```python
from build123d import *

# Parameters (mm, degrees)
CROQUIS1_W              = 33.02
CROQUIS1_H              = 10.414
SALIENTE_EXTRUIR1_DEPTH = 0.5
CROQUIS2_R              = 2.5
CROQUIS2_R_2            = 2.35
CROQUIS2_R_3            = 0.9
CROQUIS2_R_4            = 0.7
CROQUIS2_W              = 2
CROQUIS2_H              = 2
SALIENTE_EXTRUIR2_DEPTH = 0.05
CORTAR_EXTRUIR1_START   = -30.1
CROQUIS3_R              = 2.35
CROQUIS3_R_2            = 0.7
CORTAR_EXTRUIR1_DEPTH   = 30.1
CROQUIS4_R              = 0.7
CORTAR_EXTRUIR2_DEPTH   = 40.1
CROQUIS5_W              = 22.32
CROQUIS5_H              = 8.014
SALIENTE_EXTRUIR3_DEPTH = 5
CROQUIS6_W              = 4.5
CROQUIS6_H              = 6.414
CORTAR_EXTRUIR3_DEPTH   = 1.5
CROQUIS7_R              = 3.5
CORTAR_EXTRUIR4_DEPTH   = 3
C_PULA1_FACE_RADIUS     = 3.5
C_PULA1_HEIGHT          = 3
C_PULA2_FACE_RADIUS     = 3.5
C_PULA2_HEIGHT          = 3.2
CROQUIS8_R              = 0.4
SALIENTE_EXTRUIR4_DEPTH = 0.05


with BuildPart() as part:
    # Croquis1 → Saliente-Extruir1 (new, symmetric)
    with BuildSketch(Plane.XY):
        Rectangle(CROQUIS1_W, CROQUIS1_H)
    extrude(amount=SALIENTE_EXTRUIR1_DEPTH, both=True)

    # Croquis2 → Saliente-Extruir2 (add)
    # profile 1 of 5: a face of its own
    with BuildSketch(Plane.XY.offset(0.5)):
        with Locations((-12.7, 0)):
            Circle(CROQUIS2_R)
        with Locations((-12.7, 0)):
            Circle(CROQUIS2_R_2, mode=Mode.SUBTRACT)
    # profile 2 of 5: a face of its own
    with BuildSketch(Plane.XY.offset(0.5)):
        with Locations((15.01, 3.707)):
            Circle(CROQUIS2_R_3)
        with Locations((15.01, 3.707)):
            Circle(CROQUIS2_R_4, mode=Mode.SUBTRACT)
    # profile 3 of 5: a face of its own
    with BuildSketch(Plane.XY.offset(0.5)):
        with Locations((15.01, 1.207)):
            Circle(CROQUIS2_R_3)
        with Locations((15.01, 1.207)):
            Circle(CROQUIS2_R_4, mode=Mode.SUBTRACT)
    # profile 4 of 5: a face of its own
    with BuildSketch(Plane.XY.offset(0.5)):
        with Locations((15.01, -1.293)):
            Circle(CROQUIS2_R_3)
        with Locations((15.01, -1.293)):
            Circle(CROQUIS2_R_4, mode=Mode.SUBTRACT)
    # profile 5 of 5: a face of its own
    with BuildSketch(Plane.XY.offset(0.5)):
        with Locations((15.01, -3.707)):
            Rectangle(CROQUIS2_W, CROQUIS2_H)
    extrude(amount=SALIENTE_EXTRUIR2_DEPTH)

    # Croquis3 → Cortar-Extruir1 (cut)
    with BuildSketch(Plane.XY.offset(0.5).offset(CORTAR_EXTRUIR1_START)):
        with Locations((-12.7, 0)):
            Circle(CROQUIS3_R)
        with Locations((15.01, 3.707)):
            Circle(CROQUIS3_R_2)
        with Locations((15.01, 1.207)):
            Circle(CROQUIS3_R_2)
        with Locations((15.01, -1.293)):
            Circle(CROQUIS3_R_2)
    extrude(amount=CORTAR_EXTRUIR1_DEPTH, mode=Mode.SUBTRACT)

    # Croquis4 → Cortar-Extruir2 (cut)
    with BuildSketch(Plane.XY.offset(0.55)):
        with Locations((15.01, -3.707)):
            Circle(CROQUIS4_R)
    extrude(amount=-CORTAR_EXTRUIR2_DEPTH, mode=Mode.SUBTRACT)

    # Croquis5 → Saliente-Extruir3 (add)
    with BuildSketch(Plane.XY.offset(0.5)):
        with Locations((2.15, 0)):
            Rectangle(CROQUIS5_W, CROQUIS5_H)
    extrude(amount=SALIENTE_EXTRUIR3_DEPTH)

    # Croquis6 → Cortar-Extruir3 (cut)
    with BuildSketch(Plane.XY.offset(5.5)):
        with Locations((2.15, 0)):
            Rectangle(CROQUIS6_W, CROQUIS6_H)
    extrude(amount=-CORTAR_EXTRUIR3_DEPTH, mode=Mode.SUBTRACT)

    # Croquis7 → Cortar-Extruir4 (cut)
    with BuildSketch(Plane.XY.offset(5.5)):
        with Locations((-4.8, 0)):
            Circle(CROQUIS7_R)
        with Locations((9.1, 0)):
            Circle(CROQUIS7_R)
    extrude(amount=-CORTAR_EXTRUIR4_DEPTH, mode=Mode.SUBTRACT)

    # Cúpula1: a dome of height H over a round flat face of radius A is a cap of a sphere of radius (A * A + H * H) / (2 * H)
    c_pula1_r = (C_PULA1_FACE_RADIUS * C_PULA1_FACE_RADIUS + C_PULA1_HEIGHT * C_PULA1_HEIGHT) / (2 * C_PULA1_HEIGHT)
    c_pula1_base = Plane((-4.8, 0, 2.5), z_dir=(0, 0, 1))
    with Locations(c_pula1_base.offset(C_PULA1_HEIGHT - c_pula1_r)):
        c_pula1_ball = Sphere(c_pula1_r, mode=Mode.PRIVATE)
    add(split(c_pula1_ball, bisect_by=c_pula1_base, keep=Keep.TOP, mode=Mode.PRIVATE))

    # Cúpula2: a dome of height H over a round flat face of radius A is a cap of a sphere of radius (A * A + H * H) / (2 * H)
    c_pula2_r = (C_PULA2_FACE_RADIUS * C_PULA2_FACE_RADIUS + C_PULA2_HEIGHT * C_PULA2_HEIGHT) / (2 * C_PULA2_HEIGHT)
    c_pula2_base = Plane((9.1, 0, 2.5), z_dir=(0, 0, 1))
    with Locations(c_pula2_base.offset(C_PULA2_HEIGHT - c_pula2_r)):
        c_pula2_ball = Sphere(c_pula2_r, mode=Mode.PRIVATE)
    add(split(c_pula2_ball, bisect_by=c_pula2_base, keep=Keep.TOP, mode=Mode.PRIVATE))

    # Croquis8 → Saliente-Extruir4 (add)
    with BuildSketch(Plane.XY.offset(0.5)):
        with Locations((9.1, 4.417)):
            Circle(CROQUIS8_R)
        with Locations((-7.01, 4.417)):
            Circle(CROQUIS8_R)
        with Locations((-5.71, 4.417)):
            Circle(CROQUIS8_R)
        with Locations((-4.41, 4.417)):
            Circle(CROQUIS8_R)
        with Locations((-3.11, 4.417)):
            Circle(CROQUIS8_R)
        with Locations((-1.81, 4.417)):
            Circle(CROQUIS8_R)
        with Locations((-0.51, 4.417)):
            Circle(CROQUIS8_R)
        with Locations((0.79, 4.417)):
            Circle(CROQUIS8_R)
        with Locations((2.09, 4.417)):
            Circle(CROQUIS8_R)
        with Locations((3.39, 4.417)):
            Circle(CROQUIS8_R)
        with Locations((-7.01, -4.417)):
            Circle(CROQUIS8_R)
        with Locations((-5.71, -4.417)):
            Circle(CROQUIS8_R)
        with Locations((-4.41, -4.417)):
            Circle(CROQUIS8_R)
        with Locations((-3.11, -4.417)):
            Circle(CROQUIS8_R)
        with Locations((-1.81, -4.417)):
            Circle(CROQUIS8_R)
        with Locations((-0.51, -4.417)):
            Circle(CROQUIS8_R)
        with Locations((0.79, -4.417)):
            Circle(CROQUIS8_R)
        with Locations((2.09, -4.417)):
            Circle(CROQUIS8_R)
        with Locations((3.39, -4.417)):
            Circle(CROQUIS8_R)
        with Locations((9.1, -4.417)):
            Circle(CROQUIS8_R)
    extrude(amount=SALIENTE_EXTRUIR4_DEPTH)


solid = part.part
```
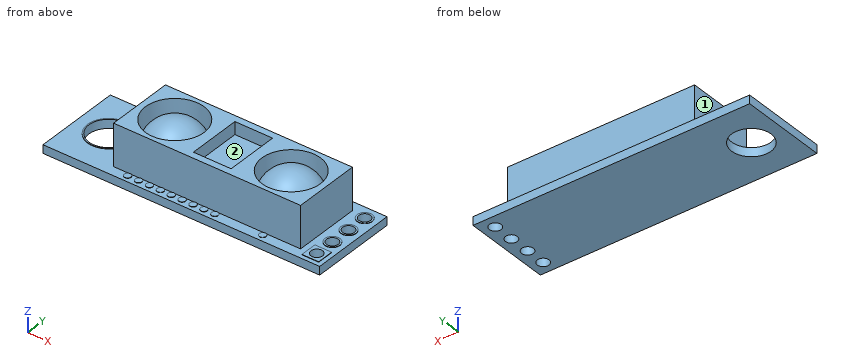
Can you work these out from the model? Positions are in its coordinate system, mm. Face numbers are marked on the shaded views. Give positions to 0.01 mm unless a question says otherwise; leave off trailing zeros. Loops run counter-clockwise (first coordinate to the right, second up) from the corner with the lowest first, then second, coordinate; pieces in that order, holes last. Notation, with made-up numbers: M 81.25,-23 L 115.25,-23 A21 cw 115.25,6 Z; hole C -31,-30.75 d10. An arc over 180 degrees is marked long. Answer in a Markdown table with one row per item.
1. Thinking about a two-plate mould opening in Y: for the marked faces 1 and 2, which applies, released by +Y, released by -Y, zero draft, split by the parting line, or undercut?
Taken from the geometry:
| item | result |
|---|---|
| face 1 | zero draft |
| face 2 | undercut |
2. Suppose I cut it at C-C on z = 3.25. Write out the boundary of the cut face in (x, y), plus the area to 3 significant figures.
Taken from the geometry:
| item | result |
|---|---|
| outline | M -9.01,-4.01 L 13.31,-4.01 L 13.31,4.01 L -9.01,4.01 Z; C -4.8,0 d6.6; C 9.1,0 d6.7; hole C -4.8,0 d7; hole C 9.1,0 d7 |
| area | 171 mm² |
3. Suppose I cut it at A-A on z = 5. Write out the boundary of the cut face in (x, y).
Taken from the geometry:
| item | result |
|---|---|
| outline | M -9.01,-4.01 L 13.31,-4.01 L 13.31,4.01 L -9.01,4.01 Z; C -4.8,0 d3.63; C 9.1,0 d4.21; hole C -4.8,0 d7; hole M -0.1,-3.21 L 4.4,-3.21 L 4.4,3.21 L -0.1,3.21 Z; hole C 9.1,0 d7 |
4. If I drill on line 1 along Y through (x, z) = (15.01, -0.25); line 2 along Y through (x, z) = (9.1, 4.65); line 3 along Y through (x, z) = (-6, 4), over which ranges is the centre line in solid material (lowest first)?
Taken from the geometry:
| item | result |
|---|---|
| line 1 | y = -5.21 to -4.41, -3.01 to -1.99, -0.59 to 0.51, 1.91 to 3.01, 4.41 to 5.21 |
| line 2 | y = -4.01 to -3.5, -2.51 to 2.51, 3.5 to 4.01 |
| line 3 | y = -4.01 to -3.29, -2.63 to 2.63, 3.29 to 4.01 |
5. For pin 1 Ø0.6 at (x, y) = (2, 4.5) entering from +Z; pin 2 Ø0.8 at (x, z) = (3, 5) entering from -Y; pin 3 Ø1.6 at (x, z) = (2, 4.5) entering from +Y, each with a flat end and sliding along its axis, tell me the tip position at first contact or that it passes through.
Taken from the geometry:
| item | result |
|---|---|
| pin 1 | stops at z = 0.55 |
| pin 2 | stops at y = -4.01 |
| pin 3 | stops at y = 4.01 |
6. Suppose I cut it at D-D on x = 15.01. Count the separate pieces of the cut face and the enclosed holes in it, plus the area to 3 significant figures.
Taken from the geometry:
| item | result |
|---|---|
| separate pieces | 5 |
| enclosed holes | 0 |
| area | 4.90 mm² |
